Verification items for the finished model (mm, model axes). A direction names the side the tool comes from. Round coordinates to 2 decimals unless told otherwise and drop trailing zeros. Order: outer loops, then holes, each group sorted by start corner. A loop starts at its lowest first (then second) coordinate and runs counter-clockwise, first axis right, second up. Notation, with made-up numbers: (49.25, 53) -> (64.25, 53) arc R25 cw to (64.25, 70) -> close; hole circle Ø6 at (69, 46.25). An arc over 180 degrees is marked (long way). Return JSON: item names as keys, results as strings. Group by question number.
Item 1: Access from +Z, -Z, +X, -X, +Y, -Y to the whole of each face (thin tool, end or side, straight path). Record for faces 1 (the flat face through (0, 40, -31)), 2 (the flat face through (-35, 40, -20)), 3 (the cylindrical face through (-0.228, 40.133, -8.965)), 4 (the cylindrical face through (-18.777, 27.32, -22.051)), 5 (the flat face through (0, 40, -8.4)).
Item 2: Depth check by flat-ended pin: pin 1 Ø9.5 at (x, y) = (15, 39.5) entering from +Z; pin 2 Ø6 at (x, y) = (-42, 71.5) entering from +Z; pin 3 Ø5 at (x, z) = (-35.5, -20.5) entering from -Y. Enter the tip coordinate at first touch or a pass-through.
Item 3: Sectioned sample at A-A on x = -20. Record the cut outline in (y, z) (3 decimals), plus the area to 3 significant figures.
Item 4: Sectioned sample at C-C on z = -19.7. Record the cut outline in (x, y) (3 decimals), plus the area to 3 significant figures.
Item 5: Draft check along Z on faces 6 (the cylindrical face through (-18.777, 51.472, -22.051)), 7 (the flat face through (0, 30.5, -20)), 8 (the cylindrical face through (-0.228, 40.133, -26.965)). Enter one of: pulls with the +Z half, pulls with the -Z half, needs draft (parallel to the pull), parting line crosses it, or undercut.
Item 6: Sectioned sample at D-D on x = -9. Record the cut outline in (y, z), plus the area to 3 significant figures.
Item 7: Scan lines: probe 1 along Z at (x, y) = (0, 40); probe 2 along Y at (x, z) = (-13, -11); probe 3 along Z at (x, y) = (21, 46). Record each from-to range of solid material in increasing order. Write a range as from..to.
Item 8: Sectioned sample at B-B on y = 36. Record the cut outline in (x, z).
```python
from build123d import *

# Parameters (mm, degrees)
SKETCH023_W       = 70
SKETCH023_H       = 19
PAD010_DEPTH      = 22.6
SKETCH001_R       = 1.75
POCKET007_DEPTH   = 19.001
SKETCH002_R       = 2.65
PAD011_DEPTH      = 4
PAD011_DEPTH_BACK = 28
SKETCH026_R       = 33.5
PAD014_DEPTH      = 25
SKETCH027_R       = 12.875
PAD015_DEPTH      = 2.55


with BuildPart() as obj1:
    # Sketch023 → Pad010 (new body)
    with BuildSketch(Plane.XY):
        Rectangle(SKETCH023_W, SKETCH023_H)
    extrude(amount=PAD010_DEPTH)

    # Sketch001 (on Face3 of Pad010) → Pocket007 (cut, through all)
    with BuildSketch(Plane.XZ.offset(9.5)):
        with Locations((0, 20.3)):
            Circle(SKETCH001_R)
        with Locations((0, 2.3)):
            Circle(SKETCH001_R)
    extrude(amount=-POCKET007_DEPTH, mode=Mode.SUBTRACT)

    # Sketch002 (on Face8 of Pocket007) → Pad011 (join, two sides)
    with BuildSketch(Plane.XZ.offset(9.5)) as pad011_sk:
        with Locations((-20, 11.3)):
            Circle(SKETCH002_R)
    extrude(amount=PAD011_DEPTH)
    extrude(pad011_sk.sketch, amount=-PAD011_DEPTH_BACK)

    # Sketch026 (on Face12 of Pad011) → Pad014 (join)
    with BuildSketch(Plane.XZ.offset(13.5)):
        with Locations((-20, 11.3)):
            Circle(SKETCH026_R)
    extrude(amount=PAD014_DEPTH)

    # Sketch027 (on Face14 of Pad014) → Pad015 (join)
    with BuildSketch(Plane(origin=(0, 18.5, 0), x_dir=(-1, 0, 0), z_dir=(0, 1, 0))):
        with Locations((20, 11.3)):
            Circle(SKETCH027_R)
    extrude(amount=-PAD015_DEPTH)


with BuildPart() as obj1_1:
    # Body002 placement: moved
    add(obj1.part.moved(Location((0, -40, -31))))


with BuildPart() as part_mirroring:
    # Part__Mirroring: instance of obj1
    add(obj1_1.part.mirror(Plane(origin=(0, 0, 0), x_dir=(1, 0, 0), z_dir=(0, 1, 0))))


solid = part_mirroring.part
```
Recorded:
{
 "1": {"face 1": "-Z, +X, -X", "face 2": "+Z, -Z, -X, -Y", "face 3": "-Y", "face 4": "none", "face 5": "+Z, +X, -X"},
 "2": {"pin 1": "z = -8.4", "pin 2": "z = 7.89", "pin 3": "y = 30.5"},
 "3": {"outline": "(21.5, -32.575) -> (24.05, -32.575) -> (24.05, -22.35) -> (30.5, -22.35) -> (30.5, -31) -> (49.5, -31) -> (49.5, -22.35) -> (53.5, -22.35) -> (53.5, -53.2) -> (78.5, -53.2) -> (78.5, 13.8) -> (53.5, 13.8) -> (53.5, -17.05) -> (49.5, -17.05) -> (49.5, -8.4) -> (30.5, -8.4) -> (30.5, -17.05) -> (24.05, -17.05) -> (24.05, -6.825) -> (21.5, -6.825) -> close", "area": "2,230 mm²"},
 "4": {"outline": "(-53.5, 53.5) -> (-22.65, 53.5) -> (-22.65, 49.5) -> (-35, 49.5) -> (-35, 30.5) -> (-22.65, 30.5) -> (-22.65, 24.05) -> (-32.875, 24.05) -> (-32.875, 21.5) -> (-7.125, 21.5) -> (-7.125, 24.05) -> (-17.35, 24.05) -> (-17.35, 30.5) -> (35, 30.5) -> (35, 49.5) -> (-17.35, 49.5) -> (-17.35, 53.5) -> (13.5, 53.5) -> (13.5, 78.5) -> (-53.5, 78.5) -> close", "area": "3,130 mm²"},
 "5": {"face 6": "parting line crosses it", "face 7": "needs draft", "face 8": "undercut"},
 "6": {"outline": "(21.5, -26.39) -> (24.05, -26.39) -> (24.05, -13.01) -> (21.5, -13.01) -> close; (30.5, -31) -> (49.5, -31) -> (49.5, -8.4) -> (30.5, -8.4) -> close; (53.5, -51.34) -> (78.5, -51.34) -> (78.5, 11.94) -> (53.5, 11.94) -> close", "area": "2,050 mm²"},
 "7": {"probe 1": "-31..-30.45, -26.95..-12.45, -8.95..-8.4", "probe 2": "21.5..24.05, 30.5..49.5, 53.5..78.5", "probe 3": "-31..-8.4"},
 "8": {"outline": "(-35, -31) -> (35, -31) -> (35, -8.4) -> (-35, -8.4) -> close; hole circle Ø3.5 at (0, -28.7); hole circle Ø3.5 at (0, -10.7)"}
}
